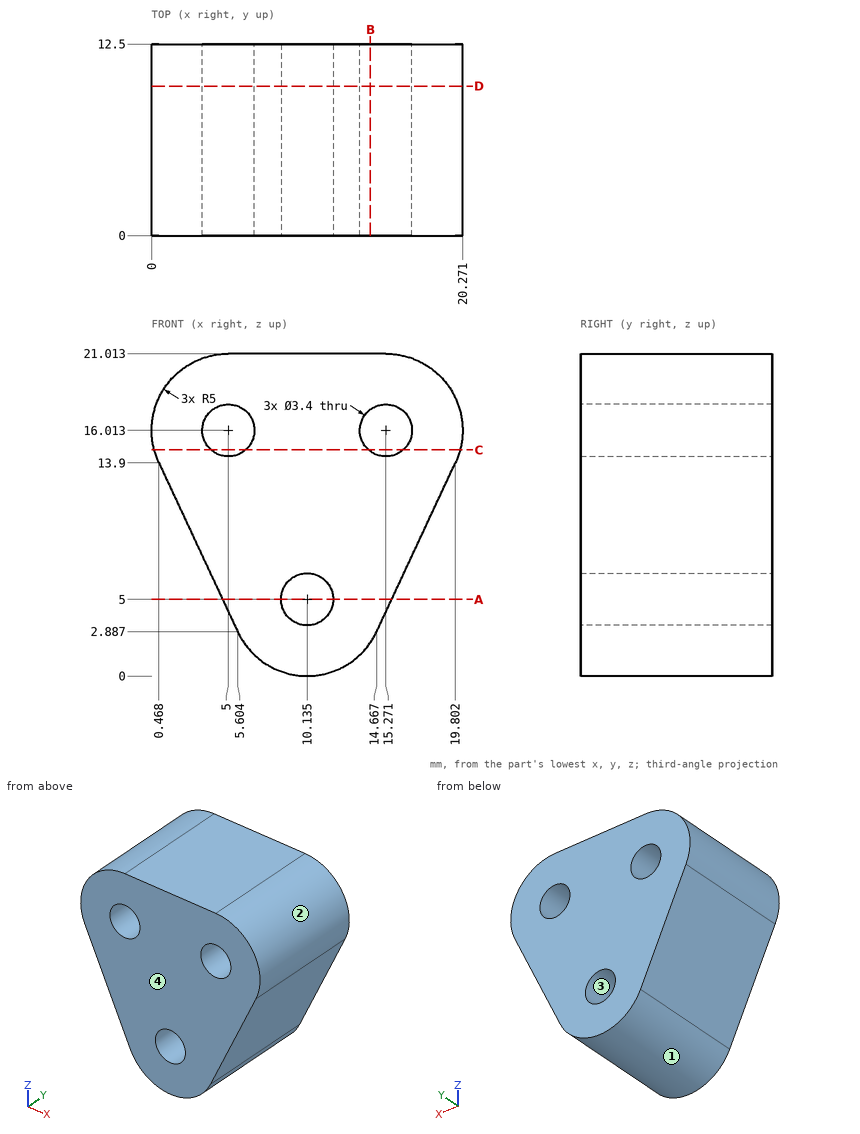
The drawing under review shows one solid part. Ordinate dimensions are in mm from its lowest x, y, z. Round coordinates to 2 decimals unless told otherwise and drop trailing zeros. Loops run counter-clockwise (first coordinate to the right, second up) from the corner with the lowest first, then second, coordinate; pieces in that order, holes last. Notation, with made-up numbers: (12, 74) -> (55, 74) arc R14 ccw to (55, 81) -> close; hole circle Ø6 at (-22, 15). An arc over 180 degrees is marked (long way). One line per question, with ' | ' between items. Start each with the question number.
Item 1: Draft analysis for pull direction Z (two halves, no side actions). For the marked faces 1, 2, 3 and 4, state which applies: +Z half, -Z half, draft (parallel to the pull), parting line (faces both ways), or undercut.
Item 2: Add section D-D, the plane y = 9.75. Write out the cut boundary in (x, z) (1 decimal).
Item 3: Wall thickness on line 1 along Z through (x, y) = (10, 10.5) (1 decimal); line 2 along Z through (x, y) = (4.25, 4) (1 decimal); line 3 along X through (y, z) = (7, 6): over which ranges is each line inside the solid? List them lowest first. Write a range as [from, to].
Item 4: For pin 1 (1.5 mm diameter, centred on y = 5.5, z = 10, fed in from +X); pin 2 (2 mm diameter, centred on x = 5, z = 16.01, fed in from +Y); pin 3 (1.5 mm diameter, centred on y = 9, z = 7, fed in from -X); pin 4 (6 mm diameter, centred on y = 5.5, z = 6.5, fed in from -X), all flat-tipped, find the tip position at first contact; note any pin that passes through.
Item 5: Add section C-C, the plane z = 14.75. Write out the cut boundary in (x, y).
Item 6: Add section B-B, the plane x = 14.25. Write out the cut boundary in (y, z).
Item 7: Add section A-A, the plane z = 5. Write out the cut boundary in (x, y) (1 decimal).
Return value:
1) face 1: -Z half | face 2: parting line | face 3: undercut | face 4: draft
2) outline: (0.5, 13.9) -> (5.6, 2.9) arc R5 ccw to (14.7, 2.9) -> (19.8, 13.9) arc R5 ccw to (15.3, 21) -> (5, 21) arc R5 ccw to start; hole circle Ø3.4 at (5, 16); hole circle Ø3.4 at (10.1, 5); hole circle Ø3.4 at (15.3, 16)
3) line 1: z = [0, 3.3], [6.7, 21] | line 2: z = [5.8, 14.5], [17.5, 21] | line 3: x = [4.15, 8.76], [11.51, 16.12]
4) pin 1: stops at x = 18.33 | pin 2: passes through | pin 3: stops at x = 3.34 | pin 4: stops at x = 2.52
5) outline: (0.16, 0) -> (3.86, 0) -> (3.86, 12.5) -> (0.16, 12.5) -> close; (6.14, 0) -> (14.13, 0) -> (14.13, 12.5) -> (6.14, 12.5) -> close; (16.41, 0) -> (20.11, 0) -> (20.11, 12.5) -> (16.41, 12.5) -> close
6) outline: (0, 2.16) -> (12.5, 2.16) -> (12.5, 14.65) -> (0, 14.65) -> close; (0, 17.37) -> (12.5, 17.37) -> (12.5, 21.01) -> (0, 21.01) -> close
7) outline: (4.6, 0) -> (8.4, 0) -> (8.4, 12.5) -> (4.6, 12.5) -> close; (11.8, 0) -> (15.7, 0) -> (15.7, 12.5) -> (11.8, 12.5) -> close
